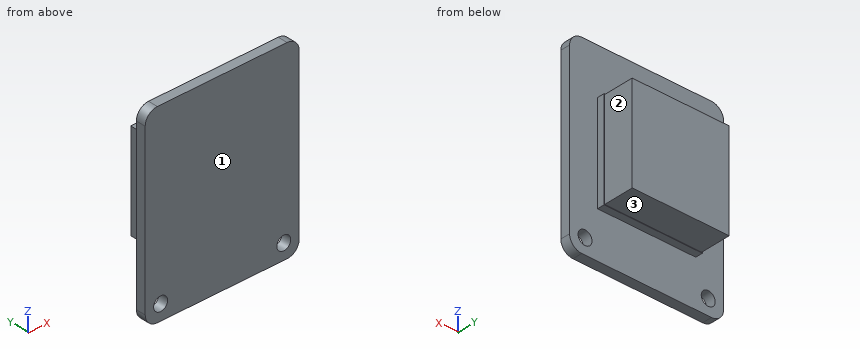
Autodesk Inventor part; units mm, degrees
ref_plane "YZ Plane" through (0, 0, 0) normal (1, 0, 0) x (0, 1, 0)
ref_plane "XZ Plane" through (0, 0, 0) normal (0, 1, 0) x (-1, 0, 0)
ref_plane "XY Plane" through (0, 0, 0) normal (0, 0, 1) x (1, 0, 0)
sketch "Boceto1" plane through (0, 0, 0) normal (0, 1, 0) x (-1, 0, 0)
  line L0 (-10.7, 15.75) -> (10.7, 15.75)
  line L1 (12.7, 13.75) -> (12.7, -13.75)
  line L2 (10.7, -15.75) -> (-10.7, -15.75)
  line L3 (-12.7, -13.75) -> (-12.7, 13.75)
  line L4 (-12.7, 15.75) -> (12.7, -15.75) construction
  line L5 (12.7, 15.75) -> (-12.7, -15.75) construction
  arc A0 (10.7, -15.75) -> (12.7, -13.75) centre (10.7, -13.75) ccw
  arc A1 (12.7, 13.75) -> (10.7, 15.75) centre (10.7, 13.75) ccw
  arc A2 (-10.7, 15.75) -> (-12.7, 13.75) centre (-10.7, 13.75) ccw
  arc A3 (-12.7, -13.75) -> (-10.7, -15.75) centre (-10.7, -13.75) ccw
  line L6 (0, -15.75) -> (0, -13.21)
  line L7 (0, -13.21) -> (10.16, -13.21)
  line L8 (0, -13.21) -> (-10.16, -13.21)
  circle A4 centre (10.16, -13.21) radius 1.15
  circle A5 centre (-10.16, -13.21) radius 1.15
  point P0 (0, 0)
  dimension "d0" = 25.4
  dimension "d1" = 31.5
  dimension "d2" = 2
  dimension "d3" = 2.54
  dimension "d4" = 10.16
  dimension "d5" = 10.16
  dimension "d6" = 2.3
  dimension "d7" = 2.3
extrude "Extrusión1" add sketch "Boceto1" along normal blind 1.6
sketch "Boceto2" plane through (0, 1.6, 0) normal (0, 1, 0) x (1, 0, 0)
  line L0 (-8, -8) -> (8, -8)
  line L1 (8, -8) -> (8, 8)
  line L2 (8, 8) -> (-8, 8)
  line L3 (-8, 8) -> (-8, -8)
  line L4 (-8, -8) -> (8, 8) construction
  line L5 (8, -8) -> (-8, 8) construction
  point P0 (0, 0)
  dimension "d10" = 16
  dimension "d11" = 16
extrude "Extrusión2" add sketch "Boceto2" along normal blind 6.2
sketch "Boceto3" plane through (0, 1.6, 0) normal (0, 1, 0) x (1, 0, 0)
  line L0 (8.1, -8.1) -> (-8.1, -8.1)
  line L1 (-8.1, -8.1) -> (-8.1, 8.1)
  line L2 (-8.1, 8.1) -> (8.1, 8.1)
  line L3 (8.1, 8.1) -> (8.1, -8.1)
  line L4 (8.1, -8.1) -> (-8.1, 8.1) construction
  line L5 (-8.1, -8.1) -> (8.1, 8.1) construction
  point P0 (0, 0)
  dimension "d14" = 16.2
  dimension "d15" = 16.2
extrude "Extrusión3" add sketch "Boceto3" along normal blind 1.2
properties part number "GPS"
For this review, take the finished solid that the model builds, in its own axes (mm). Face numbers are marked on the shaded views. A direction names the side the tool comes from. Round coordinates to 2 decimals unless told otherwise and drop trailing zeros. Write each loop counter-clockwise with the first axis right and the second up, starting at its lowest first coordinate (ties: lowest second). Pieces come first, ordered by that corner, then holes. Notation, with made-up numbers: (-27, 26) - (31, 26) arc R15 cw to (31, 42) - close; hole circle Ø3 at (65, 19). An arc over 180 degrees is marked (long way). Answer as CSV lines item,"result". Start each with the question number.
(1) For line 1 (Z direction, x = 10.16, y = 1); line 2 (X direction, y = 0.75, z = -14); line 3 (Y direction, x = -11.25, z = -7), list the stretches that pass through material, from the lowest coordinate up.
(2) Add section C-C, the plane z = 3. State the section outline as (x, y) points.
(3) Add section D-D, the plane x = -0.5. State the section outline as (y, z) points, plus the area to 3 significant figures.
(4) Add section B-B, the plane z = -13.21. State the section outline as (x, y) points, plus the area to 3 significant figures.
(5) For pin 1 (0.6 mm diameter, centred on y = 2.5, z = 0, fed in from -X); pin 2 (2.5 mm diameter, centred on x = -10.16, z = -13.21, fed in from +Y); pin 3 (2.5 mm diameter, centred on x = -2, y = 4.5, fed in from +Z), all flat-tipped, find the tip position at first contact; note any pin that passes through.
(6) Add section A-A, the plane x = 10.16. State the section outline as (y, z) points, plus the area to 3 significant figures.
(7) Machinability: for the marked faces 1, 2 and 3, which of the approach directions +Z, -Z, +X, -X, +Y, -Y give a long, thin tool a straight path to every point of the face, cutting with its end or side? Answer none if there is none.
From the geometry:
1,line 1,"z = -15.75 to -14.36, -12.06 to 15.75"
1,line 2,"x = -12.68 to -11, -9.32 to 9.32, 11 to 12.68"
1,line 3,"y = 0 to 1.6"
2,outline,"(-12.7, 0) - (12.7, 0) - (12.7, 1.6) - (8.1, 1.6) - (8.1, 2.8) - (8, 2.8) - (8, 7.8) - (-8, 7.8) - (-8, 2.8) - (-8.1, 2.8) - (-8.1, 1.6) - (-12.7, 1.6) - close"
3,outline,"(0, -15.75) - (1.6, -15.75) - (1.6, -8.1) - (2.8, -8.1) - (2.8, -8) - (7.8, -8) - (7.8, 8) - (2.8, 8) - (2.8, 8.1) - (1.6, 8.1) - (1.6, 15.75) - (0, 15.75) - close"
3,area,"150 mm²"
4,outline,"(-12.7, 0) - (-11.31, 0) - (-11.31, 1.6) - (-12.7, 1.6) - close; (-9.01, 0) - (9.01, 0) - (9.01, 1.6) - (-9.01, 1.6) - close; (11.31, 0) - (12.7, 0) - (12.7, 1.6) - (11.31, 1.6) - close"
4,area,"33.3 mm²"
5,pin 1,"stops at x = -8.1"
5,pin 2,"stops at y = 1.6"
5,pin 3,"stops at z = 8"
6,outline,"(0, -15.75) - (1.6, -15.75) - (1.6, -14.36) - (0, -14.36) - close; (0, -12.06) - (1.6, -12.06) - (1.6, 15.75) - (0, 15.75) - close"
6,area,"46.7 mm²"
7,face 1,"+Z, -Z, +X, -X, -Y"
7,face 2,"+Z, -Z, +X, +Y"
7,face 3,"-Z, +X, -X, +Y"
